```python
from build123d import *

# Parameters (mm, degrees)
F0_R      = 15.875
F1_DEPTH  = 25.4
F2_R      = 13.335
F3_DEPTH  = 22.225
F5_DEPTH  = 63.5
F6_R      = 25.4
F6_R_2    = 14.7959664705
F7_DEPTH  = 3.175
F8_R      = 2.38125
F9_DEPTH  = 25.4
F10_R     = 5.08
F12_DEPTH = 15.876
F13_SIZE  = 2.54
F14_R     = 5.08


with BuildPart() as f1:
    # F0 (on Top) → F1 (new body)
    with BuildSketch(Plane.XY):
        Circle(F0_R)
    extrude(amount=F1_DEPTH)

    # F2 (on face) → F3 (cut)
    with BuildSketch(Plane.XY.offset(25.4)):
        Circle(F2_R)
    extrude(amount=-F3_DEPTH, mode=Mode.SUBTRACT)

    # F4 (on Front) → F5 (cut, symmetric)
    with BuildSketch(Plane.XZ):
        Polygon((19.0631877631, 25.4), (-16.8183632195, 25.4), (-16.8183632195, 15.785567391), align=None)
    extrude(amount=F5_DEPTH, both=True, mode=Mode.SUBTRACT)

    # F6 (on face) → F7 (join)
    with BuildSketch(Plane(origin=(-5.0730085584, 0, 18.9327256873), x_dir=(0.9659258263, 0, 0.2588190451), z_dir=(-0.2588190451, 0, 0.9659258263))):
        with Locations((5.2519649236, 0)):
            Circle(F6_R)
        with Locations((5.2519649236, 0)):
            Circle(F6_R_2, mode=Mode.SUBTRACT)
    extrude(amount=F7_DEPTH)

    # F8 (on face) → F9 (cut)
    with BuildSketch(Plane(origin=(-5.8947590266, 0, 21.9995401858), x_dir=(0.9659258263, 0, 0.2588190451), z_dir=(-0.2588190451, 0, 0.9659258263))):
        with BuildLine():
            ThreePointArc((23.1907149236, 0), (25.5719649236, -2.38125), (27.9532149236, 0))
            ThreePointArc((27.9532149236, 0), (25.5719649236, 2.38125), (23.1907149236, 0))
        make_face()
        with Locations((-4.9080350764, 17.5976362049)):
            Circle(F8_R)
        with Locations((-4.9080350764, -17.5976362049)):
            Circle(F8_R)
    extrude(amount=-F9_DEPTH, mode=Mode.SUBTRACT)

    # F10
    f10_edges = [f1.edges().sort_by_distance(p)[0] for p in [
        (-15.875, 0, 0),
    ]]
    fillet(f10_edges, radius=F10_R)

    # F11 (on face) → F12 (cut, through all)
    with BuildSketch(Plane(origin=(-5.0730085584, 0, 18.9327256873), x_dir=(0.9659258263, 0, 0.2588190451), z_dir=(0.2588190451, 0, -0.9659258263))):
        with BuildLine():
            ThreePointArc((24.2529336259, -4.9057676704), (15.0639903014, -16.9949264796), (0, -18.908205428))
            ThreePointArc((0, -18.908205428), (-2.9619801154, -22.2901057135), (-7.4480353128, -21.9970451197))
            ThreePointArc((-7.4480353128, -21.9970451197), (17.9519648054, -21.9970453243), (30.6519649236, 0))
            ThreePointArc((30.6519649236, 0), (28.6627351357, -4.0315678707), (24.2529336259, -4.9057676704))
        make_face()
        with BuildLine():
            ThreePointArc((-7.4480353296, 21.99704511), (-20.1480350764, -9.7e-09), (-7.4480353128, -21.9970451197))
            ThreePointArc((-7.4480353128, -21.9970451197), (-9.9448603933, -18.2585376552), (-8.4970388552, -14.0024377576))
            ThreePointArc((-8.4970388552, -14.0024377576), (-14.3720858322, 0), (-8.4970388552, 14.0024377576))
            ThreePointArc((-8.4970388552, 14.0024377576), (-9.9448603946, 18.2585376456), (-7.4480353296, 21.99704511))
        make_face()
        with BuildLine():
            ThreePointArc((30.6519649236, 0), (17.951964797, 21.9970453292), (-7.4480353296, 21.99704511))
            ThreePointArc((-7.4480353296, 21.99704511), (-2.9619801244, 22.2901057172), (0, 18.908205428))
            ThreePointArc((0, 18.908205428), (15.0639903014, 16.9949264796), (24.2529336259, 4.9057676704))
            ThreePointArc((24.2529336259, 4.9057676704), (28.6627351357, 4.0315678707), (30.6519649236, 0))
        make_face()
    extrude(amount=-F12_DEPTH, mode=Mode.SUBTRACT)

    # F13
    f13_edges = [f1.edges().sort_by_distance(p)[0] for p in [
        (-15.113557, 0, 19.529371),
    ]]
    chamfer(f13_edges, length=F13_SIZE)

    # F14
    f14_edges = [f1.edges().sort_by_distance(p)[0] for p in [
        (-5.483884, -18.908205, 20.466133),
        (-13.691393, -14.002438, 18.266937),
        (-13.691393, 14.002438, 18.266937),
        (-5.483884, 18.908205, 20.466133),
        (17.942651, 4.905768, 26.743254),
        (17.942651, -4.905768, 26.743254),
    ]]
    fillet(f14_edges, radius=F14_R)


solid = f1.part
```
Geometry: final body of the model. Coordinates: model frame, mm. A direction names the side the tool comes from. Coordinates: 2 decimals unless noted, no trailing zeros. Loops run counter-clockwise (first coordinate to the right, second up) from the corner with the lowest first, then second, coordinate; pieces in that order, holes last. Notation, with made-up numbers: (63.5, 52) -> (100.5, 52) arc R23 cw to (100.5, 85) -> close; hole circle Ø9 at (80, 1). An arc over 180 degrees is marked (long way). Use a Markdown table: item, result. Add a question column.
(1) Pin query (flat end, axial travel): pin 1 Ø5 at (x, z) = (3, 20) entering from +Y; pin 2 Ø1 at (x, z) = (12.5, 9) entering from +Y; pin 3 Ø6 at (x, y) = (5, 13.5) entering from +Z. Return the tip coordinate at first contact, or that it passes through.
(2) Line query: line 1 along Y through (x, z) = (0, 8.75) (3 decimals); line 2 along Y through (x, z) = (8, 21.5). Output: solid intervals per line, ascending.
(3) Access query for faces 5 (the flat face through (-17.46, 3.47, 18.9)), 6 (the flat face through (-5.366, 15.224, 18.854)), 7 (the flat face through (0, 0, 3.175)). Directions: +Z, -Z, +X, -X, +Y, -Y. A direction counts if a zero-diameter tool reaches every point of the face in a straight line with its end or side. Return the directions, or none.
(4) Section query A-A, the plane z = 7. Return loops of the section in (x, y) (3 decimals), plus the area to 3 significant figures.
(5) Mould query, pull axis Y, two halves, no side actions, for faces 1 (the cylindrical face through (9.218, 16.907, 24.383)), 2 (the cylindrical face through (-19.36, 0.17, 16.73)), 3 (the cylindrical face through (12.719, 4.005, 11.366)), 4 (the flat face through (0, 0, 0)). Classes: pulls with the +Y half, pulls with the -Y half, needs draft (parallel to the pull), parting line crosses it, or undercut.
Answer:
| question | item | result |
|---|---|---|
| 1 | pin 1 | stops at y = 19.62 |
| 1 | pin 2 | stops at y = 10.39 |
| 1 | pin 3 | stops at z = 25.62 |
| 2 | line 1 | y = -15.875 to -13.335, 13.335 to 15.875 |
| 2 | line 2 | y = -13.71 to -10.67, 10.67 to 13.71 |
| 3 | face 5 | +Z, -X, +Y, -Y |
| 3 | face 6 | -Z |
| 3 | face 7 | +Z |
| 4 | outline | circle Ø31.75 at (0, 0); hole circle Ø26.67 at (0, 0) |
| 4 | area | 233 mm^2 |
| 5 | face 1 | pulls with the +Y half |
| 5 | face 2 | parting line crosses it |
| 5 | face 3 | undercut |
| 5 | face 4 | needs draft |
